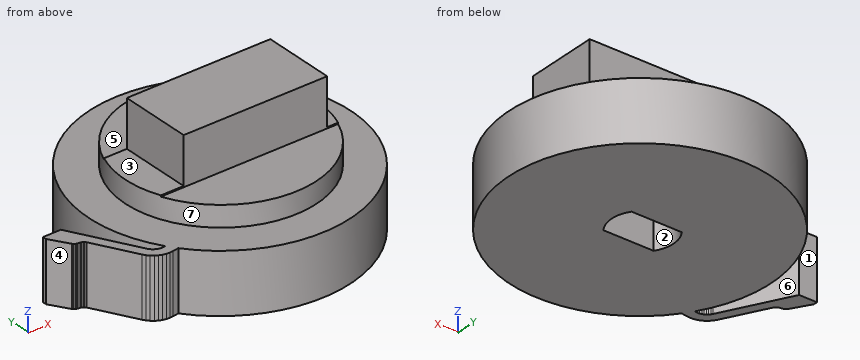
```python
from build123d import *

# Parameters (mm, degrees)
EXTRUDE001_DEPTH        = 10
BOX004_W                = 17
BOX004_H                = 16
BOX004_DEPTH            = 25
BOX005_W                = 17
BOX005_H                = 16
BOX005_DEPTH            = 25
BOX006_W                = 17
BOX006_H                = 16
BOX006_DEPTH            = 25
BOX003_W                = 17
BOX003_H                = 16
BOX003_DEPTH            = 25
CYLINDER006_R           = 8
CYLINDER006_DEPTH       = 6
EXTRUDE_DEPTH           = 5
EXTRUDE_PLACEMENT_ANGLE = 90


with BuildPart() as stepper_axis:
    # Sketch003 (on Face140 of Part__Feature) → Extrude001 (new body)
    with BuildSketch(Plane(origin=(-0.300362, -8.01257, -12.75), x_dir=(1, 0, 0), z_dir=(0, 0, 1))):
        with BuildLine():
            Line((-2.088538, 9.514445), (2.111462, 9.514445))
            ThreePointArc((2.101642, 6.522728), (2.584459, 8.017018), (2.111462, 9.514445))
            Line((-2.098358, 6.522728), (2.101642, 6.522728))
            ThreePointArc((-2.088538, 9.514445), (-2.573641, 8.020163), (-2.098358, 6.522728))
        make_face()
    extrude(amount=EXTRUDE001_DEPTH)


with BuildPart() as stepper_axis_1:
    # Extrude001 placement: moved
    add(stepper_axis.part.moved(Location((0, 0, 3))))


with BuildPart() as cube004:
    # Box004 → Box004 (new body)
    with BuildSketch(Plane(origin=(-8.5, -19, 2), x_dir=(1, 0, 0), z_dir=(0, 0, 1))):
        with Locations((8.5, 8)):
            Rectangle(BOX004_W, BOX004_H)
    extrude(amount=BOX004_DEPTH)


with BuildPart() as cube005:
    # Box005 → Box005 (new body)
    with BuildSketch(Plane(origin=(6.5, -3, 2.1), x_dir=(1, 0, 0), z_dir=(0, 0, 1))):
        with Locations((8.5, 8)):
            Rectangle(BOX005_W, BOX005_H)
    extrude(amount=BOX005_DEPTH)


with BuildPart() as cube006:
    # Box006 → Box006 (new body)
    with BuildSketch(Plane(origin=(-22.5, -12, 2.1), x_dir=(1, 0, 0), z_dir=(0, 0, 1))):
        with Locations((8.5, 8)):
            Rectangle(BOX006_W, BOX006_H)
    extrude(amount=BOX006_DEPTH)


with BuildPart() as fusion001:
    # Box003 → Box003 (new body)
    with BuildSketch(Plane(origin=(-8.5, 3, 2), x_dir=(1, 0, 0), z_dir=(0, 0, 1))):
        with Locations((8.5, 8)):
            Rectangle(BOX003_W, BOX003_H)
    extrude(amount=BOX003_DEPTH)

    # Fusion001: union Cube004, Cube005, Cube006
    add(cube004.part)
    add(cube005.part)
    add(cube006.part)


with BuildPart() as cut004:
    # Cylinder006 → Cylinder006 (new body)
    with BuildSketch(Plane.XY):
        Circle(CYLINDER006_R)
    extrude(amount=CYLINDER006_DEPTH)

    # Cut004: cut Fusion001
    add(fusion001.part, mode=Mode.SUBTRACT)


with BuildPart() as clutch_fit:
    # Sketch → Extrude (new body)
    with BuildSketch(Plane.YZ):
        with BuildLine():
            Line((76.233353, -16.168262), (76.215729, -16.28697))
            Line((76.215729, -16.28697), (76.204231, -16.437162))
            Line((76.204231, -16.437162), (76.215622, -16.589155))
            Line((76.215622, -16.589155), (76.252785, -16.739346))
            Line((76.252785, -16.739346), (76.312019, -16.88286))
            Line((76.312019, -16.88286), (76.388969, -17.011848))
            Line((76.388969, -17.011848), (76.485733, -17.129137))
            Line((76.485733, -17.129137), (76.599709, -17.23061))
            Line((76.599709, -17.23061), (76.728439, -17.313751))
            Line((76.728439, -17.313751), (82.114944, -20.238707))
            Line((82.114944, -20.238707), (82.114944, -21.732918))
            Line((82.114944, -21.732918), (81.789139, -21.729336))
            Line((81.789139, -21.729336), (80.303963, -20.801414))
            Line((80.303963, -20.801414), (80.242294, -20.755711))
            Line((80.242294, -20.755711), (80.188026, -20.701096))
            Line((80.188026, -20.701096), (80.142899, -20.638897))
            Line((80.142899, -20.638897), (80.107841, -20.570471))
            Line((80.107841, -20.570471), (80.083717, -20.497528))
            Line((80.083717, -20.497528), (80.071022, -20.421675))
            Line((80.071022, -20.421675), (80.059006, -20.286879))
            Line((80.059006, -20.286879), (80.045197, -20.206167))
            Line((80.045197, -20.206167), (80.01815, -20.128645))
            Line((80.01815, -20.128645), (79.97892, -20.056633))
            Line((79.97892, -20.056633), (79.92849, -19.992046))
            Line((79.92849, -19.992046), (79.868156, -19.936562))
            Line((79.868156, -19.936562), (79.799576, -19.891676))
            Line((79.799576, -19.891676), (76.345589, -18.015881))
            Line((76.345589, -18.015881), (76.11525, -17.86721))
            Line((76.11525, -17.86721), (75.910469, -17.684519))
            Line((75.910469, -17.684519), (75.734512, -17.473183))
            Line((75.734512, -17.473183), (75.59462, -17.237131))
            Line((75.59462, -17.237131), (75.490318, -16.982098))
            Line((75.490318, -16.982098), (75.42775, -16.714771))
            Line((75.42775, -16.714771), (75.404984, -16.441053))
            Line((75.404984, -16.441053), (75.425179, -16.167168))
            Line((75.425179, -16.167168), (75.501405, -15.659048))
            ThreePointArc((76.233353, -16.168262), (88.369051, 2.056336), (75.501405, -15.659048))
        make_face()
    extrude(amount=EXTRUDE_DEPTH)


with BuildPart() as clutch_fit_1:
    # Extrude placement: moved
    add(clutch_fit.part.moved(Location((6.886491, -82.061934, 0.254467))).rotate(Axis((6.886491, -82.061934, 0.254467), (0, 1, 0)), EXTRUDE_PLACEMENT_ANGLE))

    # Fusion002: union Cut004
    add(cut004.part)

    # Cut007: cut stepper_axis
    add(stepper_axis_1.part, mode=Mode.SUBTRACT)


with BuildPart() as clutch_fit_2:
    # Cut007 placement: moved
    add(clutch_fit_1.part.moved(Location((0, 0, 5))))


solid = clutch_fit_2.part
```
Source: CAD feature listing. Evaluate the final solid. Frame: model axes, mm. Face numbers are marked on the shaded views. A direction names the side the tool comes from. Give positions to 0.01 mm unless a question says otherwise; leave off trailing zeros. Order: outer loops, then holes, each group sorted by start corner. A loop starts at its lowest first (then second) coordinate and runs counter-clockwise, first axis right, second up.
(1) Section query A-A (y = 7.5). Return the cut outline in (x, z), plus the area to 3 significant figures.
(2) Material intervals for line 1 along Y through (x, z) = (3.5, 9.25); line 2 along Z through (x, y) = (0.25, -1); line 3 along Z through (x, y) = (-5.75, -9.25), sorted ascending.
(3) Section query B-B (y = -4.5). Return the cut outline in (x, z).
(4) Contact query for flat-ended pins moving along their axis: P1, Ø4, axis at x = 2, y = -6.5, coming from the +Z side; P2, Ø6, axis at x = 0, z = 9.5, coming from the -Y side; P3, Ø1.2, axis at y = -1.5, z = 9, coming from the +X side; P4, Ø1, axis at y = -8.5, z = 9, coming from the -X side. Output: stop coordinate, or through.
(5) Section query D-D (z = 9.5). Return the cut outline in (x, y).
(6) Access query for the marked faces 1, 2 and 3. Directions: +Z, -Z, +X, -X, +Y, -Y. A direction counts if a zero-diameter tool reaches every point of the face in a straight line with its end or side. Return the directions, or none.
(7) Pull-direction query (X, two-part tool) for the marked faces 4, 5, 6 and 7; classes: +X half, -X half, draft (parallel to the pull), parting line (faces both ways), or undercut.
(8) Section query C-C (x = 0). Return the cut outline in (y, z).
Outcome:
1. outline: (-8.07, 0.25) - (7.98, 0.25) - (7.98, 5.25) - (2.78, 5.25) - (2.78, 7) - (-2.78, 7) - (-2.78, 5.25) - (-8.07, 5.25) - close
1. area: 90.0 mm2
2. line 1: y = -3 to 3
2. line 2: z = 5.25 to 11
2. line 3: z = 0.25 to 5.25
3. outline: (-11.79, 0.25) - (-10.88, 0.25) - (-10.88, 5.25) - (-11.79, 5.25) - close; (-10, 0.25) - (9.91, 0.25) - (9.91, 5.25) - (6.61, 5.25) - (6.61, 7) - (-6.61, 7) - (-6.61, 5.25) - (-10, 5.25) - close
4. P1: stops at z = 7
4. P2: stops at y = -8
4. P3: stops at x = 6.5
4. P4: passes through
5. outline: (-5.5, -3) - (6.5, -3) - (6.5, 3) - (-5.5, 3) - close
6. face 1: +Z, -Z, -X, +Y
6. face 2: -Z
6. face 3: +Z, -X, +Y, -Y
7. face 4: -X half
7. face 5: draft
7. face 6: undercut
7. face 7: parting line
8. outline: (-10.9, 0.25) - (-1.49, 0.25) - (-1.49, 5.25) - (1.5, 5.25) - (1.5, 0.25) - (11, 0.25) - (11, 5.25) - (8, 5.25) - (8, 7) - (3, 7) - (3, 11) - (-3, 11) - (-3, 7) - (-8, 7) - (-8, 5.25) - (-10.9, 5.25) - close
